```python
from build123d import *

# Parameters (mm, degrees)
F0_R     = 2.5
F1_DEPTH = 300


with BuildPart() as f1:
    # F0 (on Top) → F1 (new body)
    with BuildSketch(Plane.XY):
        with BuildLine():
            ThreePointArc((10, 8), (9.414214, 9.414214), (8, 10))
            Line((8, 10), (3.6, 10))
            Line((3.6, 10), (3.6, 9.1))
            Line((3.6, 9.1), (3.1, 9.1))
            Line((3.1, 9.1), (3.1, 8.2))
            Line((3.1, 8.2), (5.45, 8.2))
            Line((5.45, 8.2), (5.45, 6.298528))
            Line((5.45, 6.298528), (4.579818, 5.428346))
            Line((4.579818, 5.428346), (0.25, 5.428346))
            Line((0.25, 5.428346), (0, 4.928346))
            Line((0, 4.928346), (-0.25, 5.428346))
            Line((-0.25, 5.428346), (-4.579818, 5.428346))
            Line((-4.579818, 5.428346), (-5.45, 6.298528))
            Line((-5.45, 6.298528), (-5.45, 8.2))
            Line((-5.45, 8.2), (-3.1, 8.2))
            Line((-3.1, 8.2), (-3.1, 9.1))
            Line((-3.1, 9.1), (-3.6, 9.1))
            Line((-3.6, 9.1), (-3.6, 10))
            Line((-3.6, 10), (-8, 10))
            ThreePointArc((-8, 10), (-9.414214, 9.414214), (-10, 8))
            Line((-10, 8), (-10, 3.6))
            Line((-10, 3.6), (-9.1, 3.6))
            Line((-9.1, 3.6), (-9.1, 3.1))
            Line((-9.1, 3.1), (-8.2, 3.1))
            Line((-8.2, 3.1), (-8.2, 5.45))
            Line((-8.2, 5.45), (-6.298528, 5.45))
            Line((-6.298528, 5.45), (-5.428346, 4.579818))
            Line((-5.428346, 4.579818), (-5.428346, 0.25))
            Line((-5.428346, 0.25), (-4.928346, 0))
            Line((-4.928346, 0), (-5.428346, -0.25))
            Line((-5.428346, -0.25), (-5.428346, -4.579818))
            Line((-5.428346, -4.579818), (-6.298528, -5.45))
            Line((-6.298528, -5.45), (-8.2, -5.45))
            Line((-8.2, -5.45), (-8.2, -3.1))
            Line((-8.2, -3.1), (-9.1, -3.1))
            Line((-9.1, -3.1), (-9.1, -3.6))
            Line((-9.1, -3.6), (-10, -3.6))
            Line((-10, -3.6), (-10, -8))
            ThreePointArc((-10, -8), (-9.414214, -9.414214), (-8, -10))
            Line((-8, -10), (-3.6, -10))
            Line((-3.6, -10), (-3.6, -9.1))
            Line((-3.6, -9.1), (-3.1, -9.1))
            Line((-3.1, -9.1), (-3.1, -8.2))
            Line((-3.1, -8.2), (-5.45, -8.2))
            Line((-5.45, -8.2), (-5.45, -6.298528))
            Line((-5.45, -6.298528), (-4.579818, -5.428346))
            Line((-4.579818, -5.428346), (-0.25, -5.428346))
            Line((-0.25, -5.428346), (0, -4.928346))
            Line((0, -4.928346), (0.25, -5.428346))
            Line((0.25, -5.428346), (4.579818, -5.428346))
            Line((4.579818, -5.428346), (5.45, -6.298528))
            Line((5.45, -6.298528), (5.45, -8.2))
            Line((5.45, -8.2), (3.1, -8.2))
            Line((3.1, -8.2), (3.1, -9.1))
            Line((3.1, -9.1), (3.6, -9.1))
            Line((3.6, -9.1), (3.6, -10))
            Line((3.6, -10), (8, -10))
            ThreePointArc((8, -10), (9.414214, -9.414214), (10, -8))
            Line((10, -8), (10, -3.6))
            Line((10, -3.6), (9.1, -3.6))
            Line((9.1, -3.6), (9.1, -3.1))
            Line((9.1, -3.1), (8.2, -3.1))
            Line((8.2, -3.1), (8.2, -5.45))
            Line((8.2, -5.45), (6.298528, -5.45))
            Line((6.298528, -5.45), (5.428346, -4.579818))
            Line((5.428346, -4.579818), (5.428346, -0.25))
            Line((5.428346, -0.25), (4.928346, 0))
            Line((4.928346, 0), (5.428346, 0.25))
            Line((5.428346, 0.25), (5.428346, 4.579818))
            Line((5.428346, 4.579818), (6.298528, 5.45))
            Line((6.298528, 5.45), (8.2, 5.45))
            Line((8.2, 5.45), (8.2, 3.1))
            Line((8.2, 3.1), (9.1, 3.1))
            Line((9.1, 3.1), (9.1, 3.6))
            Line((9.1, 3.6), (10, 3.6))
            Line((10, 3.6), (10, 8))
        make_face()
        Circle(F0_R, mode=Mode.SUBTRACT)
    extrude(amount=F1_DEPTH)


solid = f1.part
```
Here's how the part is built. I have some questions about the finished solid (model axes, mm). Give positions to 0.01 mm unless a question says otherwise; leave off trailing zeros. Use one line per item in the form item = value. Start each with the question number.
Q1. Thinking about a two-plate mould opening in Y: for faces 1 (the cylindrical face through (-0.54, -2.44, 147.9)), 2 (the flat face through (-2, 2, 300)), which applies, +Y half, -Y half, draft (parallel to the pull), parting line (faces both ways), or undercut?
Q2. Will these pins go through, and if not, where does the flat tip stop? pin 1 Ø0.5 at (y, z) = (-8.5, 222.5) entering from +X; pin 2 Ø3 at (x, z) = (-0.5, 185.5) entering from -Y; pin 3 Ø3 at (x, z) = (-2, 237) entering from -Y.
Q3. I need wall thicknesses on line 1 along X through (y, z) = (-4, 247); line 2 along X through (y, z) = (3.5, 162). Which ranges of each line are inside material? Lowest first, please.
Taken from the geometry:
q1.face_1 = undercut
q1.face_2 = draft
q2.pin_1 = 9.98
q2.pin_2 = -5.43
q2.pin_3 = -9.1
q3.line_1 = -10 to -8.2, -5.43 to 5.43, 8.2 to 10
q3.line_2 = -9.1 to -8.2, -5.43 to 5.43, 8.2 to 9.1
